Part model, mm, in its own coordinate system. Face numbers are marked on the shaded views. Round coordinates to 2 decimals unless told otherwise and drop trailing zeros. Loops run counter-clockwise (first coordinate to the right, second up) from the corner with the lowest first, then second, coordinate; pieces in that order, holes last. Notation, with made-up numbers: M 37.5,29 L 65.5,29 A15 ccw 65.5,44 Z; hole C 50.5,-11.75 d11. An arc over 180 degrees is marked long. Write each question's results on one line, items separated by ' | '.
from build123d import *

# Parameters (mm, degrees)
F0_R          = 25
F0_R_2        = 5
F1_DEPTH      = 10
F1_DEPTH_BACK = 10
F2_W          = 70
F2_H          = 10
F3_ANGLE_BACK = 45
F3_ANGLE      = 90
F4_COUNT      = 3
F4_ANGLE      = 240
F6_R          = 4.99999


# Not quite as in the source:
# - a fillet or chamfer is up to 0.001 mm smaller than in the source, because OpenCascade refuses the exact size


with BuildPart() as f1:
    # F0 (on Top) → F1 (new body, two sides)
    with BuildSketch(Plane.XY) as f1_sk:
        with BuildLine():
            ThreePointArc((25.282899435, -16.1485292259), (28.7965881924, -8.4116888004), (30, 0))
            ThreePointArc((30, 0), (28.8728814443, 8.1459632398), (25.5762188598, 15.6798287247))
            ThreePointArc((25.5762188598, 15.6798287247), (15.2387828621, 25.8414298537), (1.3435868258, 29.969897805))
            ThreePointArc((1.3435868258, 29.969897805), (-14.7599432924, 26.1178880081), (-26.3672394325, 14.3097409029))
            ThreePointArc((-26.3672394325, 14.3097409029), (-29.9987261544, 0.2764581545), (-26.6264862609, -13.8213685791))
            ThreePointArc((-26.6264862609, -13.8213685791), (-15.2387828621, -25.8414298537), (0.7910205727, -29.9895696277))
            ThreePointArc((0.7910205727, -29.9895696277), (14.7599432924, -26.1178880081), (25.282899435, -16.1485292259))
        make_face()
        Circle(F0_R, mode=Mode.SUBTRACT)
        with BuildLine():
            ThreePointArc((1.3435868258, 29.969897805), (15.2387828621, 25.8414298537), (25.5762188598, 15.6798287247))
            Line((25.5762188598, 15.6798287247), (31.7810181804, 39.6262733222))
            ThreePointArc((31.7810181804, 39.6262733222), (27.9793762729, 48.5939196708), (18.3333577354, 47.2428132348))
            Line((18.3333577354, 47.2428132348), (1.3435868258, 29.969897805))
        make_face()
        with Locations((24.0367650986, 41.6328984003)):
            Circle(F0_R_2, mode=Mode.SUBTRACT)
        with BuildLine():
            Line((31.7467975399, -39.4985601529), (25.282899435, -16.1485292259))
            ThreePointArc((25.282899435, -16.1485292259), (14.7599432924, -26.1178880081), (0.7910205727, -29.9895696277))
            Line((0.7910205727, -29.9895696277), (18.4268502641, -47.3363057635))
            ThreePointArc((18.4268502641, -47.3363057635), (28.0938807679, -48.5278104698), (31.7467975399, -39.4985601529))
        make_face()
        with Locations((24.0367650986, -41.6328984003)):
            Circle(F0_R_2, mode=Mode.SUBTRACT)
        with BuildLine():
            ThreePointArc((-26.6264862609, -13.8213685791), (-29.9987261544, 0.2764581545), (-26.3672394325, 14.3097409029))
            Line((-26.3672394325, 14.3097409029), (-50.2078684445, 7.7100324413))
            ThreePointArc((-50.2078684445, 7.7100324413), (-56.0732570408, -0.066109201), (-50.0801552753, -7.7442530819))
            Line((-50.0801552753, -7.7442530819), (-26.6264862609, -13.8213685791))
        make_face()
        with Locations((-48.0735301971, 0)):
            Circle(F0_R_2, mode=Mode.SUBTRACT)
    extrude(amount=F1_DEPTH)
    extrude(f1_sk.sketch, amount=-F1_DEPTH_BACK)


with BuildPart() as f3:
    # F2 (on Front) → F3 (revolve)
    with BuildSketch(Plane.XZ, mode=Mode.PRIVATE) as f3_sk:
        with Locations((-34.9688172646, 0)):
            Rectangle(F2_W, F2_H)
    revolve(f3_sk.sketch.rotate(Axis((0.0311827354, 0, 0), (0, 0, -1)), -F3_ANGLE_BACK), axis=Axis((0.0311827354, 0, 0), (0, 0, -1)), revolution_arc=F3_ANGLE)


with BuildPart() as f4_1:
    # F4: instance of F3
    add(f3.part.rotate(Axis((0, 0, 10), (0, 0, -1)), 1 * F4_ANGLE / (F4_COUNT - 1)))


with BuildPart() as f4_2:
    # F4: instance of F3
    add(f3.part.rotate(Axis((0, 0, 10), (0, 0, -1)), 2 * F4_ANGLE / (F4_COUNT - 1)))


with BuildPart() as f1_1:
    add(f1.part)

    # F5: cut F3, F4_1, F4_2
    add(f3.part, mode=Mode.SUBTRACT)
    add(f4_1.part, mode=Mode.SUBTRACT)
    add(f4_2.part, mode=Mode.SUBTRACT)

    # F6 (radius 5 in the source; OpenCascade refuses exactly that, so slightly less here)
    f6_edges = [f1_1.edges().sort_by_distance(p)[0] for p in [
        (26.568658, 7.096223, 5),
        (26.568658, 7.096223, -5),
        (26.568658, -7.096223, -5),
        (26.568658, -7.096223, 5),
        (-7.13882, -26.557245, 5),
        (-7.13882, -26.557245, -5),
        (-19.429839, 19.461022, -5),
        (-7.13882, 26.557245, -5),
        (-19.429839, 19.461022, 5),
        (-7.13882, 26.557245, 5),
        (-19.429839, -19.461022, -5),
        (-19.429839, -19.461022, 5),
    ]]
    fillet(f6_edges, radius=F6_R)


solid = f1_1.part
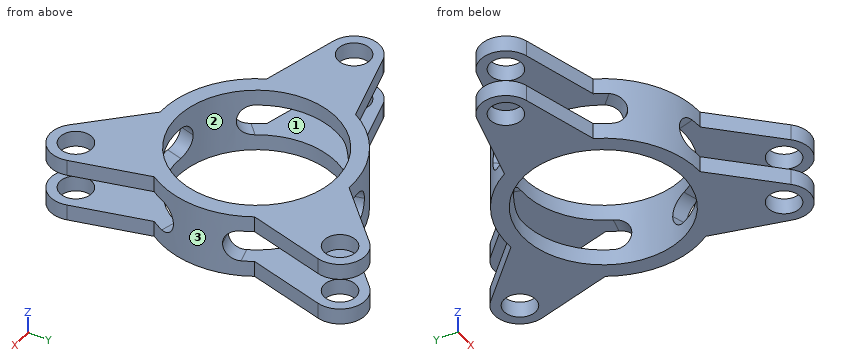
Item 1: Band-saw the part on B-B on x = 21. Count the separate pieces of the cut face and the enclosed holes in it, and give its area (3 significant figures).
Filled sheet:
separate pieces: 8 | enclosed holes: 0 | area: 551 mm^2
Item 2: Two-plate mould, pull along X, no slides. Class the marked faces 1, 2 and 3: +X half, -X half, draft (parallel to the pull), parting line (faces both ways), or undercut.
Filled sheet:
face 1: draft | face 2: undercut | face 3: +X half
Item 3: Band-saw the part on D-D on x = 10. Give the cut face in (y, z).
Filled sheet:
outline: M -39.05,-10 L -22.91,-10 L -22.91,-5 L -39.05,-5 Z; M -39.05,5 L -22.91,5 L -22.91,10 L -39.05,10 Z; M 22.91,-10 L 38.77,-10 L 38.77,-5 L 22.91,-5 Z; M 22.91,5 L 38.77,5 L 38.77,10 L 22.91,10 Z
Item 4: Band-saw the part on A-A on y = 0. Give the cut face in (x, z).
Filled sheet:
outline: M -56.07,-10 L -53.07,-10 L -53.07,-5 L -56.07,-5 Z; M -56.07,5 L -53.07,5 L -53.07,10 L -56.07,10 Z; M -43.07,-10 L -25,-10 L -25,-5 L -43.07,-5 Z; M -43.07,5 L -25,5 L -25,10 L -43.07,10 Z; M 25,-10 L 30,-10 L 30,10 L 25,10 Z
Item 5: Band-saw the part on C-C on z = -2.25. Give the cut face in (x, y), and give its area (3 significant figures).
Filled sheet:
outline: M -21.57,-20.85 A30 ccw -7.27,-29.11 L -5.97,-24.28 A25 cw -18.04,-17.31 Z; M -21.57,20.85 L -18.04,17.31 A25 cw -5.97,24.28 L -7.27,29.11 A30 ccw Z; M 24.01,-6.96 L 28.84,-8.26 A30 ccw 28.84,8.26 L 24.01,6.96 A25 cw Z | area: 231 mm^2
Item 6: Drop flat-ended pins along their axis: P1, Ø3, axis at x = -22.5, z = -5, coming from the +Y side; P2, Ø9, axis at x = 24.04, y = -41.63, coming from the -Z side; P3, Ø4, axis at y = -35.5, z = -7.5, coming from the +X side; P4, Ø1, axis at y = 21.5, z = 5, coming from the +X side. Give the stop position or say it passes through.
Filled sheet:
P1: y = 21.42 | P2: through | P3: x = 31.19 | P4: x = 27.21
Item 7: Wall check: L1, parallel to Z at x = -44.5, y = 8; L2, parallel to Y at x = -13, z = -8.5; L3, parallel to Y at x = -14, z = -3. Give the ranges that are in metal, low to high.
Filled sheet:
L1: -10 to -5, 5 to 10 | L2: -27.04 to -21.35, 21.35 to 27.04 | L3: -26.53 to -20.71, 20.71 to 26.53
